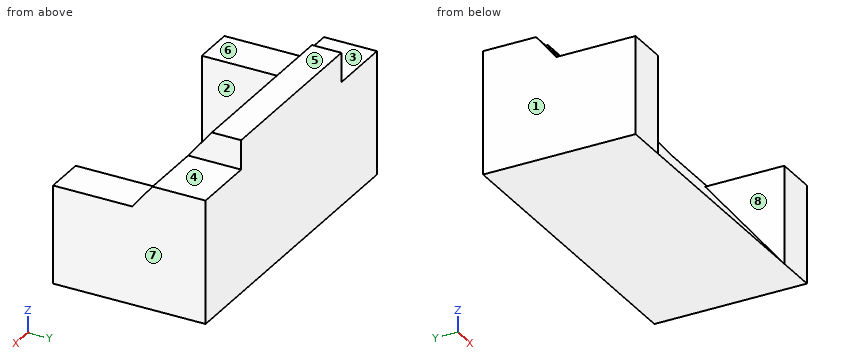
from build123d import *

# Parameters (mm, degrees)
PAD_DEPTH      = 26.5
PAD_DEPTH_BACK = 26.5
SKETCH001_W    = 5
SKETCH001_H    = 11
POCKET_DEPTH   = 10
SKETCH002_W    = 16.7
SKETCH002_H    = 7
PAD001_DEPTH   = 26


with BuildPart() as part:
    # Sketch → Pad (new body, two sides)
    with BuildSketch(Plane.YZ) as pad_sk:
        Polygon((-24.544346, 1.192678), (-50.544346, 1.192678), (-29.544346, 27.192678), (-24.544346, 27.192678), align=None)
    extrude(amount=PAD_DEPTH)
    extrude(pad_sk.sketch, amount=-PAD_DEPTH_BACK)

    # Sketch001 (on Face4 of Pad) → Pocket (cut)
    with BuildSketch(Plane.ZX.offset(-24.544346)):
        with Locations((24.692678, 21)):
            Rectangle(SKETCH001_W, SKETCH001_H)
    pocket = extrude(amount=-POCKET_DEPTH, mode=Mode.SUBTRACT)

    # Mirrored: Pocket across Sketch001 H_Axis
    add(pocket.mirror(Plane(origin=(0, -24.544346, 0), x_dir=(0, 1, 0), z_dir=(1, 0, 0))), mode=Mode.SUBTRACT)

    # Sketch002 (on Face2 of Mirrored) → Pad001 (join)
    with BuildSketch(Plane.ZX.offset(-24.544346)):
        with Locations((9.542678, 23)):
            Rectangle(SKETCH002_W, SKETCH002_H)
    pad001 = extrude(amount=-PAD001_DEPTH)

    # Mirrored001: Pad001 across Sketch002 H_Axis
    add(pad001.mirror(Plane(origin=(0, -24.544346, 0), x_dir=(0, 1, 0), z_dir=(1, 0, 0))))


solid = part.part
Input: part model. Units: mm. Frame: model coordinates. Face numbers are marked on the shaded views. A direction names the side the tool comes from. Coordinates: 2 decimals unless noted, no trailing zeros. Order: outer loops, then holes, each group sorted by start corner. A loop starts at its lowest first (then second) coordinate and runs counter-clockwise, first axis right, second up.
1. Ray query, line 1 along X through (y, z) = (-39.5, 17.5); line 2 along Z through (x, y) = (8, -35.75); line 3 along Z through (x, y) = (-17, -32.75). Return the intervals inside material, ascending.
Checked values:
line 1: x = -26.5 to -19.5, 19.5 to 26.5
line 2: z = 1.19 to 19.51
line 3: z = 1.19 to 22.19
2. Cut plane A-A, the plane y = -27. Return loops of the section in (x, z).
Checked values:
outline: (-26.5, 1.19) - (26.5, 1.19) - (26.5, 22.19) - (15.5, 22.19) - (15.5, 27.19) - (-15.5, 27.19) - (-15.5, 22.19) - (-26.5, 22.19) - close
3. Access query for the marked faces 4, 5, 6, 7 and 8. Directions: +Z, -Z, +X, -X, +Y, -Y. A direction counts if a zero-diameter tool reaches every point of the face in a straight line with its end or side. Return the directions, or none.
Checked values:
face 4: +Z, +X, +Y, -Y
face 5: +Z, +X, -X, +Y, -Y
face 6: +Z, +X, -X, -Y
face 7: +Z, -Z, +X, +Y, -Y
face 8: +Z, -Y
4. Contact query for flat-ended pins moving along their axis: P1, Ø5.5, axis at x = 22, y = -44, coming from the +Z side; P2, Ø5.5, axis at y = -30, z = 24, coming from the -X side; P3, Ø2.5, axis at x = -19, y = -31, coming from the +Z side; P4, Ø1, axis at x = -16.5, z = 15, coming from the -Y side. Output: stop coordinate, or through.
Checked values:
P1: stops at z = 17.89
P2: stops at x = -26.5
P3: stops at z = 22.19
P4: stops at y = -39.8
5. Cut plane C-C, the plane x = -17.5. Return loops of the section in (y, z), plus the area to 3 significant figures.
Checked values:
outline: (-50.54, 1.19) - (-24.54, 1.19) - (-24.54, 22.19) - (-33.58, 22.19) - close
area: 368 mm2
6. Cut plane D-D, the plane x = 8.5. Return loops of the section in (y, z).
Checked values:
outline: (-50.54, 1.19) - (-24.54, 1.19) - (-24.54, 27.19) - (-29.54, 27.19) - close
7. Cut plane B-B, the plane z = 17. Return loops of the section in (x, y).
Checked values:
outline: (-26.5, -50.54) - (-19.5, -50.54) - (-19.5, -37.78) - (19.5, -37.78) - (19.5, -50.54) - (26.5, -50.54) - (26.5, -24.54) - (-26.5, -24.54) - close
8. Draft query along X for the marked faces 1, 2 and 3. Return one class per face: +X half, -X half, draft (parallel to the pull), parting line (faces both ways), or undercut.
Checked values:
face 1: -X half
face 2: undercut
face 3: draft
